Geometry check sheet. Reference: the model listing, model coordinates, mm. A direction names the side the tool comes from. Give positions to 0.01 mm unless a question says otherwise; leave off trailing zeros. Loops run counter-clockwise (first coordinate to the right, second up) from the corner with the lowest first, then second, coordinate; pieces in that order, holes last. Notation, with made-up numbers: (77.25, -15.75) - (90.25, -15.75) arc R20 ccw to (90.25, -1.75) - close; hole circle Ø8 at (15.25, 81). An arc over 180 degrees is marked (long way). One line per question, with ' | ' between items. Start each with the question number.
from build123d import *

# Parameters (mm, degrees)
CHAMFER_1_SIZE = 1
CHAMFER_2_SIZE = 0.5


with BuildPart() as part:
    # Эскиз1 → Повернуть1 (revolve)
    with BuildSketch(Plane.XY, mode=Mode.PRIVATE) as revolve_1_sk:
        Polygon((7, 21.5), (2, 21.5), (2, 11), (7, 11), (7, 7.5), (0, 7.5), (0, 24), (7, 24), align=None)
    revolve(revolve_1_sk.sketch.rotate(Axis((0, 0, 0), (1, 0, 0)), 90), axis=Axis((0, 0, 0), (1, 0, 0)))

    # Фаска1
    chamfer_1_edges = [part.edges().sort_by_distance(p)[0] for p in [
        (0, 0, -24),
    ]]
    chamfer(chamfer_1_edges, length=CHAMFER_1_SIZE)

    # Фаска2
    chamfer_2_edges = [part.edges().sort_by_distance(p)[0] for p in [
        (7, 0, -7.5),
        (0, 0, -7.5),
    ]]
    chamfer(chamfer_2_edges, length=CHAMFER_2_SIZE)


solid = part.part
(1) Material ranges on line 1 (Y direction, x = 4.4, z = 0); line 2 (Z direction, x = 3.25, y = -2); line 3 (Z direction, x = 5, y = -5.5), recorded low to high.
(2) Mould release check, pull along Z, two halves, no side actions. Record for faces 3 (the face through (4.465, -21.317, -2.799)), 4 (the face through (4.04, -7.21, 22.89)), 5 (the face through (7, 8, -2)): pulls with the +Z half, pulls with the -Z half, needs draft (parallel to the pull), parting line crosses it, or undercut.
(3) Tool access check on faces 1 (the face through (4.54, 10.74, -2.38)), 2 (the face through (3.458, -6.324, 4.032)). Record the directions out of +Z, -Z, +X, -X, +Y, -Y that give a thin tool (end or side, any length) a straight path to the whole face; none if there is none.
(4) Depth check by flat-ended pin: pin 1 Ø1 at (x, y) = (5, 7.5) entering from +Z; pin 2 Ø1 at (y, z) = (6.5, -15) entering from +X; pin 3 Ø4 at (x, y) = (2, -11.5) entering from +Z; pin 4 Ø3 at (y, z) = (0, 5.5) entering from +X. Enter the tip coordinate at first touch or a pass-through.
(5) Section check A-A, the plane y = 0. Record the boundary of the cut face in (x, z), and give its area (4 significant figures).
(6) Section check C-C, the plane x = 4.5. Record the boundary of the cut face in (y, z), and give its area (3 significant figures).
Numbers:
1) line 1: -24 to -21.5, -11 to -7.5, 7.5 to 11, 21.5 to 24 | line 2: -23.92 to -21.41, -10.82 to -7.23, 7.23 to 10.82, 21.41 to 23.92 | line 3: -23.36 to -20.78, -9.53 to -5.1, 5.1 to 9.53, 20.78 to 23.36
2) face 3: undercut | face 4: parting line crosses it | face 5: needs draft
3) face 1: +X | face 2: +X, -X
4) pin 1: z = 22.96 | pin 2: x = 2 | pin 3: z = 22.04 | pin 4: through
5) outline: (0, -23) - (1, -24) - (7, -24) - (7, -21.5) - (2, -21.5) - (2, -11) - (7, -11) - (7, -8) - (6.5, -7.5) - (0.5, -7.5) - (0, -8) - close; (0, 8) - (0.5, 7.5) - (6.5, 7.5) - (7, 8) - (7, 11) - (2, 11) - (2, 21.5) - (7, 21.5) - (7, 24) - (1, 24) - (0, 23) - close | area: 124.5 mm^2
6) outline: circle Ø48 at (0, 0); circle Ø22 at (0, 0); hole circle Ø43 at (0, 0); hole circle Ø15 at (0, 0) | area: 561 mm^2
